Here's the drawing with two shaded views (mm, measured from the low corner). I have some questions. Give positions to 0.01 mm unless a question says otherwise; leave off trailing zeros. Loops run counter-clockwise (first coordinate to the right, second up) from the corner with the lowest first, then second, coordinate; pieces in that order, holes last. Notation, with made-up numbers: (89.5, -30.5) - (123.5, -30.5) arc R4 cw to (123.5, -25.5) - close; hole circle Ø5 at (88.5, 8). An arc over 180 degrees is marked (long way). Use one line per item in the form item = value.
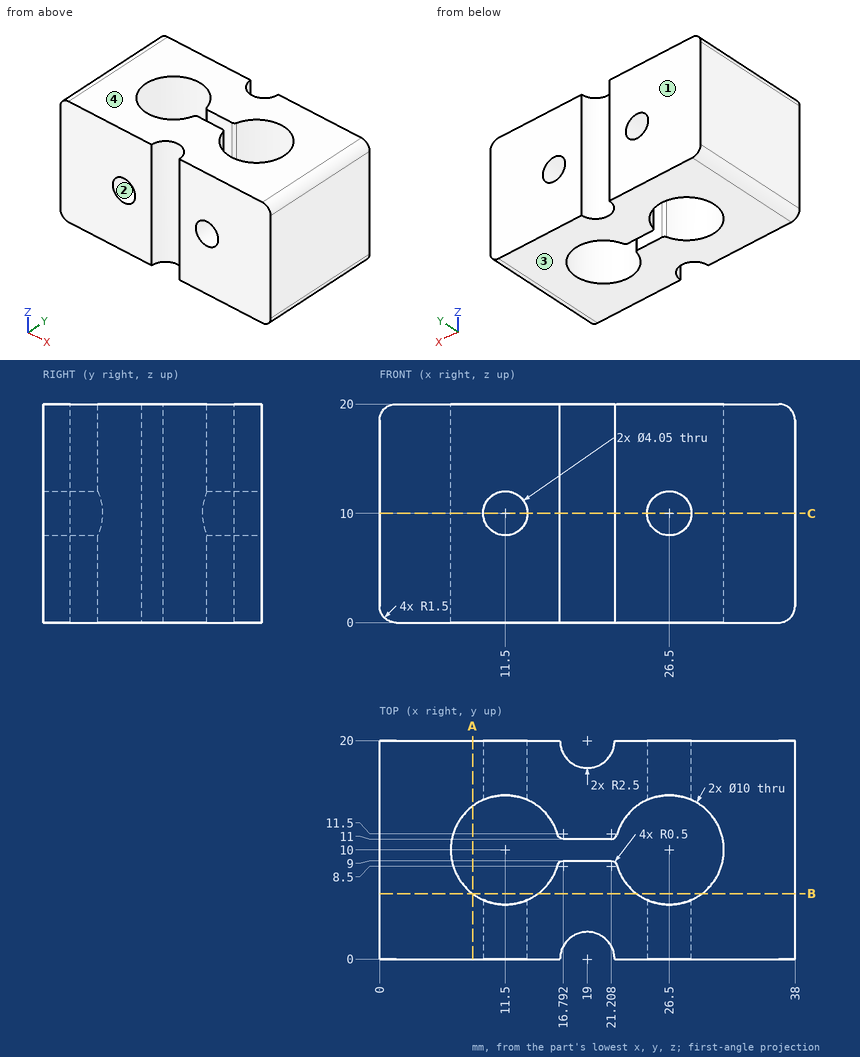
(1) If we section it at B-B (y = 6): List the corners of the cut face in (x, z) for me.
Geometry says:
outline = (0, 1.5) arc R1.5 ccw to (1.5, 0) - (8.5, 0) - (8.5, 20) - (1.5, 20) arc R1.5 ccw to (0, 18.5) - close; (14.5, 0) - (23.5, 0) - (23.5, 20) - (14.5, 20) - close; (29.5, 0) - (36.5, 0) arc R1.5 ccw to (38, 1.5) - (38, 18.5) arc R1.5 ccw to (36.5, 20) - (29.5, 20) - close
(2) If we section it at C-C (z = 10): Give the number of separate pieces and of enclosed holes in the cut face, plus the area to 3 significant figures.
Geometry says:
separate_pieces = 4
enclosed_holes = 0
area = 490 mm²
(3) For P1, Ø1.3, axis at x = 19.5, z = 9.5, coming from the -Y side; P2, Ø1.3, axis at x = 18, z = 13.5, coming from the +Y side; P3, Ø6.5, axis at x = 26.5, z = 10, coming from the +Y side, each with a flat end and sliding along its axis, tell me the tip position at first contact or that it passes through.
Geometry says:
P1 = 2.22
P2 = 18.12
P3 = 20
(4) If I drill on probe 1 along Z at (x, y) = (11.5, 1.85) (1 decimal); probe 2 along X at (y, z) = (12, 11.25); probe 3 along X at (y, z) = (14.75, 9.5), over which ranges is the centre line in solid material (lowest first)?
Geometry says:
probe_1 = 0 to 8, 12 to 20
probe_2 = 0 to 6.92, 16.08 to 21.92, 31.08 to 38
probe_3 = 0 to 9.54, 13.46 to 24.54, 28.46 to 38
(5) If we section it at A-A (x = 8.5): List the corners of the cut face in (y, z) for me.
Geometry says:
outline = (0, 0) - (6, 0) - (6, 20) - (0, 20) - close; (14, 0) - (20, 0) - (20, 20) - (14, 20) - close
(6) Thinking about a two-plate mould opening in Z: for the marked faces 1, 2, 3 and 4, which applies, pulls with the +Z half, pulls with the -Z half, needs draft (parallel to the pull), parting line crosses it, or undercut?
Geometry says:
face_1 = needs draft
face_2 = undercut
face_3 = pulls with the -Z half
face_4 = pulls with the +Z half
